Design review of the part built by this model. Coordinates are the model's own, in mm. A direction names the side the tool comes from. Round coordinates to 2 decimals unless told otherwise and drop trailing zeros. Write each loop counter-clockwise with the first axis right and the second up, starting at its lowest first coordinate (ties: lowest second). Pieces come first, ordered by that corner, then holes. Notation, with made-up numbers: M 82,-11 L 92,-11 A19 cw 92,21 Z; hole C -3,-28.5 d4. An arc over 180 degrees is marked long. Use CSV: the item, a comma, the result in double quotes.
from build123d import *

# Parameters (mm, degrees)
SKETCH1_W               = 85
SKETCH1_H               = 60
BOSS_EXTRUDE1_DEPTH     = 15
SKETCH2_W               = 20
SKETCH2_H               = 60
BOSS_EXTRUDE2_DEPTH     = 5
CUT_EXTRUDE1_DEPTH      = 106.118980208
CUT_EXTRUDE1_DEPTH_BACK = 106.118980208
SKETCH3_R               = 2.6
CUT_EXTRUDE2_START      = 15
SKETCH4_R               = 5
CUT_EXTRUDE2_DEPTH      = 5
FILLET1_R               = 1.5
CUT_EXTRUDE3_DEPTH      = 106.118980208
CUT_EXTRUDE3_DEPTH_BACK = 106.118980208
SKETCH5_R               = 4.1
CUT_EXTRUDE4_START      = 15
SKETCH6_R               = 7.5
CUT_EXTRUDE4_DEPTH      = 10
CHAMFER1_SIZE           = 3


with BuildPart() as part:
    # Sketch1 → Boss-Extrude1 (new body)
    with BuildSketch(Plane.XY):
        with Locations((-42.5, 30)):
            Rectangle(SKETCH1_W, SKETCH1_H)
    extrude(amount=BOSS_EXTRUDE1_DEPTH)

    # Sketch2 → Boss-Extrude2 (add)
    with BuildSketch(Plane.XY):
        with Locations((-10, 30)):
            Rectangle(SKETCH2_W, SKETCH2_H)
    extrude(amount=-BOSS_EXTRUDE2_DEPTH)

    # Sketch3 → Cut-Extrude1 (cut, two sides: drawn at the far end of the back side and taken through both)
    with BuildSketch(Plane.XY.offset(-CUT_EXTRUDE1_DEPTH_BACK)):
        with Locations((-10, 40)):
            Circle(SKETCH3_R)
        with Locations((-10, 20)):
            Circle(SKETCH3_R)
    extrude(amount=CUT_EXTRUDE1_DEPTH + CUT_EXTRUDE1_DEPTH_BACK, mode=Mode.SUBTRACT)

    # Sketch4 → Cut-Extrude2 (cut)
    with BuildSketch(Plane.XY.offset(CUT_EXTRUDE2_START)):
        with Locations((-10, 40)):
            Circle(SKETCH4_R)
        with Locations((-10, 20)):
            Circle(SKETCH4_R)
    extrude(amount=-CUT_EXTRUDE2_DEPTH, mode=Mode.SUBTRACT)

    # Fillet1
    fillet1_edges = [part.edges().sort_by_distance(p)[0] for p in [
        (-20, 30, -5),
        (0, 30, -5),
    ]]
    fillet(fillet1_edges, radius=FILLET1_R)

    # Sketch5 → Cut-Extrude3 (cut, two sides: drawn at the far end of the back side and taken through both)
    with BuildSketch(Plane.XY.offset(-CUT_EXTRUDE3_DEPTH_BACK)):
        with Locations((-55, 45)):
            Circle(SKETCH5_R)
        with Locations((-55, 15)):
            Circle(SKETCH5_R)
    extrude(amount=CUT_EXTRUDE3_DEPTH + CUT_EXTRUDE3_DEPTH_BACK, mode=Mode.SUBTRACT)

    # Sketch6 → Cut-Extrude4 (cut)
    with BuildSketch(Plane.XY.offset(CUT_EXTRUDE4_START)):
        with Locations((-55, 45)):
            Circle(SKETCH6_R)
        with Locations((-55, 15)):
            Circle(SKETCH6_R)
    extrude(amount=-CUT_EXTRUDE4_DEPTH, mode=Mode.SUBTRACT)

    # Chamfer1
    chamfer1_edges = [part.edges().sort_by_distance(p)[0] for p in [
        (-42.5, 60, 15),
        (-85, 30, 15),
        (-42.5, 0, 15),
        (-85, 0, 7.5),
        (-85, 60, 7.5),
        (0, 30, 15),
    ]]
    chamfer(chamfer1_edges, length=CHAMFER1_SIZE)


solid = part.part
1) The part is to be moulded in two halves that separate along Y. For faces 1 (the face through (-53, 30, 0)), 2 (the face through (-42, 58, 14)), 3 (the face through (-51.8, 11.8, 5)), say which applies: released by +Y, released by -Y, zero draft, split by the parting line, or undercut.
Answers:
face 1,"zero draft"
face 2,"released by +Y"
face 3,"undercut"
2) Add section A-A on z = 4. Write out the cut boundary in (x, y).
Answers:
outline,"M -85,3 L -82,0 L 0,0 L 0,60 L -82,60 L -85,57 Z; hole C -55,15 d8.2; hole C -55,45 d8.2; hole C -10,20 d5.2; hole C -10,40 d5.2"
3) Machinability: for faces 4 (the face through (-56.63, 37.68, 10.07)), 5 (the face through (-20, 30, -2)), 6 (the face through (0, 30, 4)), which of the approach directions +Z, -Z, +X, -X, +Y, -Y give a long, thin tool a straight path to every point of the face, cutting with its end or side? Answer none if there is none.
Answers:
face 4,"+Z"
face 5,"-Z, -X, +Y, -Y"
face 6,"+Z, -Z, +X, +Y, -Y"
4) For pin 1 Ø10.5 at (x, y) = (-55, 45) entering from -Z; pin 2 Ø4 at (y, z) = (31, -2.5) entering from -X; pin 3 Ø9 at (x, y) = (-10, 20) entering from +Z, all flat-tipped, find the tip position at first contact; note any pin that passes through.
Answers:
pin 1,"z = 0"
pin 2,"x = -20"
pin 3,"z = 10"
5) Wall thickness on line 1 along Y through (x, z) = (-10, 5.5); line 2 along X through (y, z) = (40, 1.75); line 3 along Y through (x, z) = (-55, 12): over which ranges is each line inside the solid? List them lowest first. Write a range as [from, to].
Answers:
line 1,"[0, 17.4], [22.6, 37.4], [42.6, 60]"
line 2,"[-85, -12.6], [-7.4, 0]"
line 3,"[0, 7.5], [22.5, 37.5], [52.5, 60]"
6) Add section D-D on y = 40. Write out the cut boundary in (x, z), then the cut area to 3 significant figures.
Answers:
outline,"M -85,0 L -20,0 L -20,-3.5 A1.5 ccw -18.5,-5 L -12.6,-5 L -12.6,10 L -15,10 L -15,15 L -49.41,15 L -49.41,5 L -60.59,5 L -60.59,15 L -82,15 L -85,12 Z; M -7.4,-5 L -1.5,-5 A1.5 ccw 0,-3.5 L 0,12 L -3,15 L -5,15 L -5,10 L -7.4,10 Z"
area,"1,130 mm²"
7) Add section C-C on y = 27.5. Write out the cut boundary in (x, z), then the cut area to 3 significant figures.
Answers:
outline,"M -85,0 L -20,0 L -20,-3.5 A1.5 ccw -18.5,-5 L -1.5,-5 A1.5 ccw 0,-3.5 L 0,12 L -3,15 L -82,15 L -85,12 Z"
area,"1,370 mm²"
8) Add section B-B on x = -55. Write out the cut boundary in (y, z), then the cut area to 3 significant figures.
Answers:
outline,"M 0,0 L 10.9,0 L 10.9,5 L 7.5,5 L 7.5,15 L 3,15 L 0,12 Z; M 19.1,0 L 40.9,0 L 40.9,5 L 37.5,5 L 37.5,15 L 22.5,15 L 22.5,5 L 19.1,5 Z; M 49.1,0 L 60,0 L 60,12 L 57,15 L 52.5,15 L 52.5,5 L 49.1,5 Z"
area,"509 mm²"
